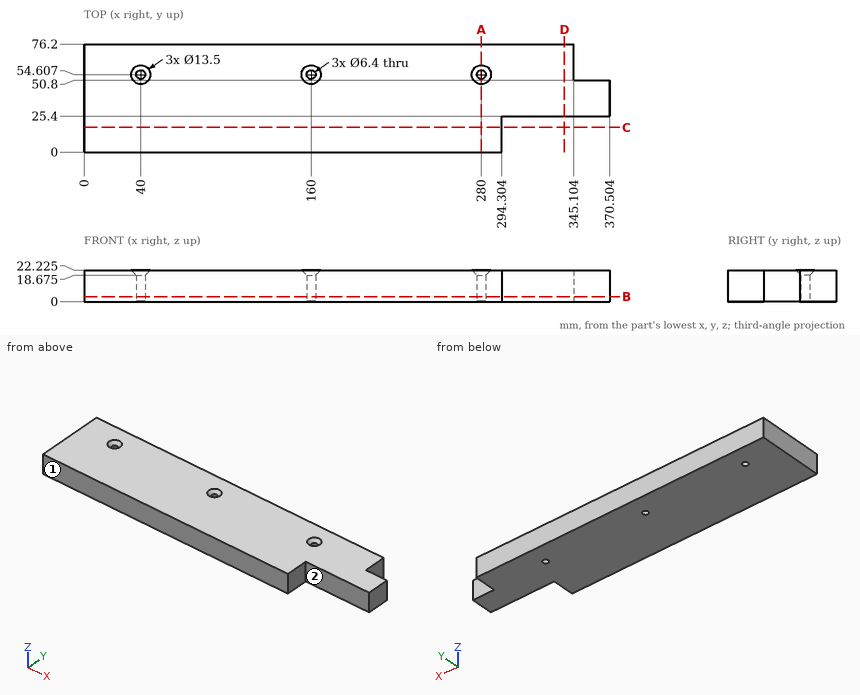
Answer from the drawing. Dimensions are ordinates in mm from the lowest x, y and z of the part. A direction names the side the tool comes from. Coordinates: 2 decimals unless noted, no trailing zeros. Order: outer loops, then holes, each group sorted by start corner. A loop starts at its lowest first (then second) coordinate and runs counter-clockwise, first axis right, second up. Notation, with made-up numbers: (-36, 36) - (-9, 36) arc R14 cw to (-9, 61) - close; hole circle Ø8 at (-22.75, 25.5). An arc over 180 degrees is marked (long way). Put each result on its own line as item: value. Start each with the question number.
1) Find section B-B (z = 3.5). Give the vertices of the cut face in (x, y) (1 decimal).
2) Find section C-C (y = 17.5). Give the vertices of the cut face in (x, z) (1 decimal), plus the area to 3 significant figures.
3) For the marked faces 1 and 2, determine the directions among +Z, -Z, +X, -X, +Y, -Y from which every point of the face is accessible in a straight line to the end or side of a thin tool.
4) Find section A-A (x = 280). Give the vertices of the cut face in (y, z) (1 decimal).
5) Flat-ended cylindrical pins translate along their axes: pin 1 (11 mm diameter, centred on y = 69, z = 10, fed in from +X); pin 2 (3 mm diameter, centred on x = 274.5, y = 37.5, fed in from -Z); pin 3 (6.5 mm diameter, centred on y = 17.5, z = 6, fed in from +X); pin 4 (11 mm diameter, centred on x = 363, z = 6, fed in from +Y). Find the tip coordinate at first contact, or state that the pin passes through.
6) Find the intervals of material crossed by line 1 (Y direction, x = 280, z = 11.5); line 2 (X direction, y = 56, z = 9.5) (1 decimal); line 3 (X direction, y = 56.5, z = 1) (1 decimal), in increasing order. Write a range as from..to.
7) Find section D-D (x = 338.5). Give the vertices of the cut face in (y, z) (1 decimal), plus the area to 3 significant figures.
Results list:
1. outline: (0, 0) - (294.3, 0) - (294.3, 25.4) - (370.5, 25.4) - (370.5, 50.8) - (345.1, 50.8) - (345.1, 76.2) - (0, 76.2) - close; hole circle Ø6.4 at (40, 54.6); hole circle Ø6.4 at (160, 54.6); hole circle Ø6.4 at (280, 54.6)
2. outline: (0, 0) - (294.3, 0) - (294.3, 22.2) - (0, 22.2) - close
2. area: 6,540 mm^2
3. face 1: +Z, -Z, +X, -X, -Y
3. face 2: +Z, -Z, +X, -Y
4. outline: (0, 0) - (51.4, 0) - (51.4, 18.7) - (47.9, 22.2) - (0, 22.2) - close; (57.8, 0) - (76.2, 0) - (76.2, 22.2) - (61.4, 22.2) - (57.8, 18.7) - close
5. pin 1: stops at x = 345.1
5. pin 2: stops at z = 0
5. pin 3: stops at x = 294.3
5. pin 4: stops at y = 50.8
6. line 1: y = 0..51.41, 57.81..76.2
6. line 2: x = 0..37.1, 42.9..157.1, 162.9..277.1, 282.9..345.1
6. line 3: x = 0..37.4, 42.6..157.4, 162.6..277.4, 282.6..345.1
7. outline: (25.4, 0) - (76.2, 0) - (76.2, 22.2) - (25.4, 22.2) - close
7. area: 1,130 mm^2
